Print and shaded views of the part. All mm, measured from the part's lowest x, y and z. A direction names the side the tool comes from. Round coordinates to 2 decimals unless told otherwise and drop trailing zeros. Loops run counter-clockwise (first coordinate to the right, second up) from the corner with the lowest first, then second, coordinate; pieces in that order, holes last. Notation, with made-up numbers: (38, -15) -> (96, -15) arc R14 cw to (96, -1) -> close; hole circle Ø6 at (8.5, -23.5). An arc over 180 degrees is marked (long way). Answer as CSV lines item,"result".
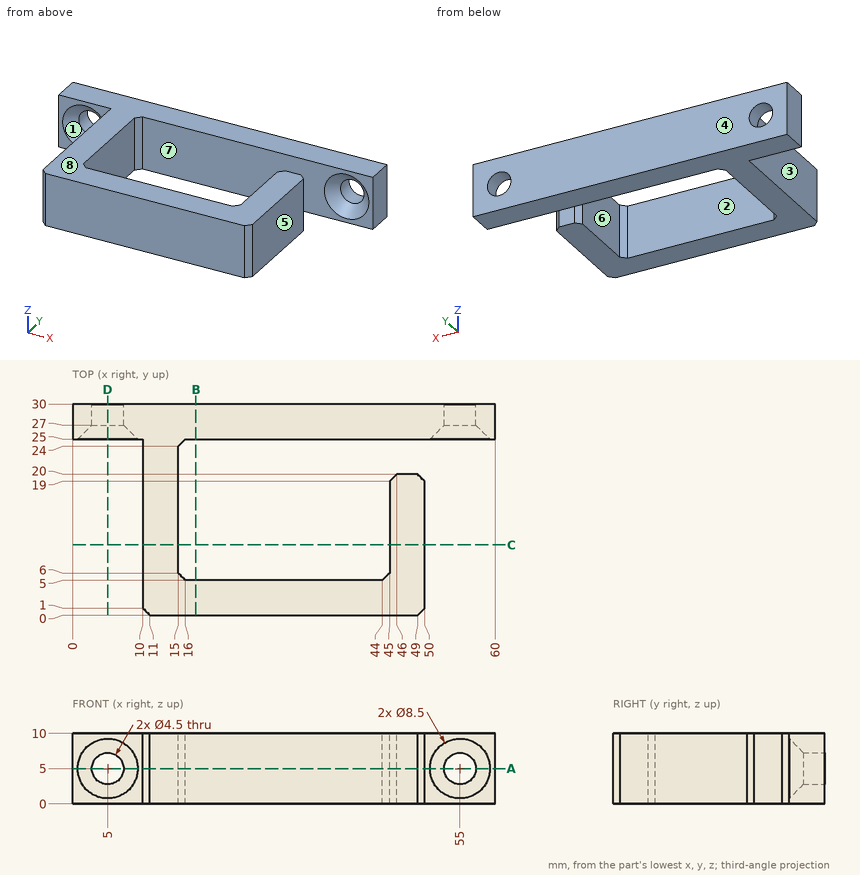
Q1. Drop flat-ended pins along their axis: P1, Ø5, axis at x = 55, z = 5, coming from the +Y side; P2, Ø4, axis at y = 14, z = 8.5, coming from the -X side; P3, Ø5, axis at y = 13, z = 7.5, coming from the +X side. Give the stop position or say it passes through.
Geometry results:
P1,"y = 30"
P2,"x = 10"
P3,"x = 50"
Q2. Saw through at D-D, the plane x = 5. Write the cut outline in (y, z), then the cut area to 3 significant figures.
Geometry results:
outline,"(25, 0) -> (30, 0) -> (30, 2.75) -> (27, 2.75) -> (25, 0.75) -> close; (25, 9.25) -> (27, 7.25) -> (30, 7.25) -> (30, 10) -> (25, 10) -> close"
area,"23.5 mm2"
Q3. Two-plate mould, pull along Y, no slides. Class the marked faces 1, 2, 3 and 4: pulls with the +Y half, pulls with the -Y half, needs draft (parallel to the pull), parting line crosses it, or undercut.
Geometry results:
face 1,"pulls with the -Y half"
face 2,"undercut"
face 3,"needs draft"
face 4,"pulls with the +Y half"
Q4. Which spindle directions (+Z, -Z, +X, -X, +Y, -Y) get a long thin tool onto all of the face, cutting with end or side? Do the marked faces 5, 6, 7 and 8. Say none if no direction does.
Geometry results:
face 5,"+Z, -Z, +X, -Y"
face 6,"+Z, -Z"
face 7,"+Z, -Z, +X"
face 8,"+Z, +X, -X, +Y, -Y"
Q5. Saw through at B-B, the plane x = 17.5. Write the cut outline in (y, z).
Geometry results:
outline,"(0, 0) -> (5, 0) -> (5, 10) -> (0, 10) -> close; (25, 0) -> (30, 0) -> (30, 10) -> (25, 10) -> close"
Q6. Saw through at C-C, the plane y = 10. Write the cut outline in (x, z).
Geometry results:
outline,"(10, 0) -> (15, 0) -> (15, 10) -> (10, 10) -> close; (45, 0) -> (50, 0) -> (50, 10) -> (45, 10) -> close"
Q7. Saw through at A-A, the plane z = 5. Give the number of separate pieces and of enclosed holes in the cut face, then the cut area to 4 significant figures.
Geometry results:
separate pieces,"3"
enclosed holes,"0"
area,"621.5 mm2"
Q8. Drill centre lines: line 1 along X through (y, z) = (28.25, 5); line 2 along Y through (x, z) = (32, 6.25); line 3 along X through (y, z) = (25.75, 5.25). Where is each one in solid material? Low to high.
Geometry results:
line 1,"0 to 2.75, 7.25 to 52.75, 57.25 to 60"
line 2,"0 to 5, 25 to 30"
line 3,"0 to 1.51, 8.49 to 51.51, 58.49 to 60"
